from build123d import *

# Parameters (mm, degrees)
BOSS_EXTRUDE1_DEPTH = 13
BOSS_EXTRUDE3_DEPTH = 0.5


with BuildPart() as part:
    # Sketch1 → Boss-Extrude1 (new body)
    with BuildSketch(Plane.XY):
        with BuildLine():
            Line((128.676424344, 77.084775656), (128.676424344, -12.915224344))
            ThreePointArc((128.676424344, -12.915224344), (125.747492156, -19.986292156), (118.676424344, -22.915224344))
            Line((118.676424344, -22.915224344), (-1.323575656, -22.915224344))
            ThreePointArc((-1.323575656, -22.915224344), (-8.394643467, -19.986292156), (-11.323575656, -12.915224344))
            Line((-11.323575656, -12.915224344), (-11.323575656, 77.084775656))
            ThreePointArc((-11.323575656, 77.084775656), (-8.394643467, 84.155843467), (-1.323575656, 87.084775656))
            Line((-1.323575656, 87.084775656), (118.676424344, 87.084775656))
            ThreePointArc((118.676424344, 87.084775656), (125.747492156, 84.155843467), (128.676424344, 77.084775656))
        make_face()
    extrude(amount=BOSS_EXTRUDE1_DEPTH)

    # Sketch10 → Boss-Extrude3 (add)
    with BuildSketch(Plane(origin=(0, 0, 0), x_dir=(-1, 0, 0), z_dir=(0, 0, -1))):
        with BuildLine():
            Line((-121.176424344, 74.084775656), (-120.176424344, 74.084775656))
            ThreePointArc((-120.176424344, 74.084775656), (-116.994443829, 75.40279514), (-115.676424344, 78.584775656))
            Line((-115.676424344, 78.584775656), (-115.676424344, 79.584775656))
            ThreePointArc((-115.676424344, 79.584775656), (-114.35840486, 82.766756171), (-111.176424344, 84.084775656))
            Line((-111.176424344, 84.084775656), (-6.176424344, 84.084775656))
            ThreePointArc((-6.176424344, 84.084775656), (-2.994443829, 82.766756171), (-1.676424344, 79.584775656))
            Line((-1.676424344, 79.584775656), (-1.676424344, 78.584775656))
            ThreePointArc((-1.676424344, 78.584775656), (-0.35840486, 75.40279514), (2.823575656, 74.084775656))
            Line((2.823575656, 74.084775656), (3.823575656, 74.084775656))
            ThreePointArc((3.823575656, 74.084775656), (7.005556171, 72.766756171), (8.323575656, 69.584775656))
            Line((8.323575656, 69.584775656), (8.323575656, -5.415224344))
            ThreePointArc((8.323575656, -5.415224344), (7.005556171, -8.59720486), (3.823575656, -9.915224344))
            Line((3.823575656, -9.915224344), (2.823575656, -9.915224344))
            ThreePointArc((2.823575656, -9.915224344), (-0.35840486, -11.233243829), (-1.676424344, -14.415224344))
            Line((-1.676424344, -14.415224344), (-1.676424344, -15.415224344))
            ThreePointArc((-1.676424344, -15.415224344), (-2.994443829, -18.59720486), (-6.176424344, -19.915224344))
            Line((-6.176424344, -19.915224344), (-111.176424344, -19.915224344))
            ThreePointArc((-111.176424344, -19.915224344), (-114.35840486, -18.59720486), (-115.676424344, -15.415224344))
            Line((-115.676424344, -15.415224344), (-115.676424344, -14.415224344))
            ThreePointArc((-115.676424344, -14.415224344), (-116.994443829, -11.233243829), (-120.176424344, -9.915224344))
            Line((-120.176424344, -9.915224344), (-121.176424344, -9.915224344))
            ThreePointArc((-121.176424344, -9.915224344), (-124.35840486, -8.59720486), (-125.676424344, -5.415224344))
            Line((-125.676424344, -5.415224344), (-125.676424344, 69.584775656))
            ThreePointArc((-125.676424344, 69.584775656), (-124.35840486, 72.766756171), (-121.176424344, 74.084775656))
        make_face()
        with BuildLine():
            Line((-121.176424344, 73.084775656), (-120.176424344, 73.084775656))
            ThreePointArc((-120.176424344, 73.084775656), (-116.287337048, 74.695688359), (-114.676424344, 78.584775656))
            Line((-114.676424344, 78.584775656), (-114.676424344, 79.584775656))
            ThreePointArc((-114.676424344, 79.584775656), (-113.651298079, 82.05964939), (-111.176424344, 83.084775656))
            Line((-111.176424344, 83.084775656), (-6.176424344, 83.084775656))
            ThreePointArc((-6.176424344, 83.084775656), (-3.70155061, 82.05964939), (-2.676424344, 79.584775656))
            Line((-2.676424344, 79.584775656), (-2.676424344, 78.584775656))
            ThreePointArc((-2.676424344, 78.584775656), (-1.065511641, 74.695688359), (2.823575656, 73.084775656))
            Line((2.823575656, 73.084775656), (3.823575656, 73.084775656))
            ThreePointArc((3.823575656, 73.084775656), (6.29844939, 72.05964939), (7.323575656, 69.584775656))
            Line((7.323575656, 69.584775656), (7.323575656, -5.415224344))
            ThreePointArc((7.323575656, -5.415224344), (6.29844939, -7.890098079), (3.823575656, -8.915224344))
            Line((3.823575656, -8.915224344), (2.823575656, -8.915224344))
            ThreePointArc((2.823575656, -8.915224344), (-1.065511641, -10.526137048), (-2.676424344, -14.415224344))
            Line((-2.676424344, -14.415224344), (-2.676424344, -15.415224344))
            ThreePointArc((-2.676424344, -15.415224344), (-3.70155061, -17.890098079), (-6.176424344, -18.915224344))
            Line((-6.176424344, -18.915224344), (-111.176424344, -18.915224344))
            ThreePointArc((-111.176424344, -18.915224344), (-113.651298079, -17.890098079), (-114.676424344, -15.415224344))
            Line((-114.676424344, -15.415224344), (-114.676424344, -14.415224344))
            ThreePointArc((-114.676424344, -14.415224344), (-116.287337048, -10.526137048), (-120.176424344, -8.915224344))
            Line((-120.176424344, -8.915224344), (-121.176424344, -8.915224344))
            ThreePointArc((-121.176424344, -8.915224344), (-123.651298079, -7.890098079), (-124.676424344, -5.415224344))
            Line((-124.676424344, -5.415224344), (-124.676424344, 69.584775656))
            ThreePointArc((-124.676424344, 69.584775656), (-123.651298079, 72.05964939), (-121.176424344, 73.084775656))
        make_face(mode=Mode.SUBTRACT)
    extrude(amount=BOSS_EXTRUDE3_DEPTH)


solid = part.part
Geometry check sheet. Reference: the model listing, model coordinates, mm. A direction names the side the tool comes from. Coordinates: 2 decimals unless noted, no trailing zeros. Order: outer loops, then holes, each group sorted by start corner. A loop starts at its lowest first (then second) coordinate and runs counter-clockwise, first axis right, second up. Notation, with made-up numbers: (9, -12.75) -> (36, -12.75) arc R16 cw to (36, 16.25) -> close; hole circle Ø7 at (-2, -1.75). An arc over 180 degrees is marked (long way). Use a Markdown table: item, result. Add a question column.
1. Set-up check for faces 1 (the face through (-6.97, 72.8, -0.25)), 2 (the face through (0.323, -11.198, -0.246)), 3 (the face through (1.11, 74.74, -0.25)), 4 (the face through (124.323, -8.632, -0.246)): record each of +Z, -Z, +X, -X, +Y, -Y from which the full face is reachable in a straight line by a thin tool's end or side.
2. Mould release check, pull along Y, two halves, no side actions. Record for faces 5 (the face through (117, 75.4, -0.2)), 6 (the face through (114.323, -18.632, -0.246)), 7 (the face through (116.245, -10.569, -0.246)): pulls with the +Y half, pulls with the -Y half, needs draft (parallel to the pull), parting line crosses it, or undercut.
3. Material ranges on L1, parallel to Z at x = 71, y = 12.5, recorded low to high.
4. Cross-section at A-A (x = 15.5). Enter the section's corners in (y, z), and give its area (3 significant figures).
5. Go/stop test with flat-tipped pins: pin 1 Ø0.6 at (y, z) = (79, 0) entering from -X; pin 2 Ø0.6 at (x, z) = (120.5, -0.5) entering from -Y; pin 3 Ø4 at (x, y) = (111.5, 62.5) entering from -Z. Record where each tip stops, or that it passes through.
6. Cross-section at B-B (y = 44.5). Enter the section's corners in (x, z), and give its area (3 significant figures).
Filled sheet:
| question | item | result |
|---|---|---|
| 1 | face 1 | -Z, -X, +Y |
| 1 | face 2 | -Z, -X, -Y |
| 1 | face 3 | -Z |
| 1 | face 4 | -Z, +X, -Y |
| 2 | face 5 | pulls with the +Y half |
| 2 | face 6 | pulls with the -Y half |
| 2 | face 7 | undercut |
| 3 | L1 | 0 to 13 |
| 4 | outline | (-22.92, 0) -> (-19.92, 0) -> (-19.92, -0.5) -> (-18.92, -0.5) -> (-18.92, 0) -> (83.08, 0) -> (83.08, -0.5) -> (84.08, -0.5) -> (84.08, 0) -> (87.08, 0) -> (87.08, 13) -> (-22.92, 13) -> close |
| 4 | area | 1,430 mm2 |
| 5 | pin 1 | x = -11.19 |
| 5 | pin 2 | y = -9.92 |
| 5 | pin 3 | z = 0 |
| 6 | outline | (-11.32, 0) -> (-8.32, 0) -> (-8.32, -0.5) -> (-7.32, -0.5) -> (-7.32, 0) -> (124.68, 0) -> (124.68, -0.5) -> (125.68, -0.5) -> (125.68, 0) -> (128.68, 0) -> (128.68, 13) -> (-11.32, 13) -> close |
| 6 | area | 1,820 mm2 |
